```python
from build123d import *

# Parameters (mm, degrees)
EXTRUDE_1_DEPTH      = 5
EXTRUDE_1_DEPTH_BACK = 5
SKETCH_2_R           = 1.2
CUT_EXTRUDE_1_DEPTH  = 6
SKETCH_3_R           = 1.2
CUT_EXTRUDE_2_DEPTH  = 6
FILLET_1_R           = 1
FILLET_2_R           = 2
CUT_EXTRUDE1_DEPTH   = 2
CUT_EXTRUDE2_DEPTH   = 2


with BuildPart() as part:
    # Sketch 1 → Extrude 1 (new body, two sides)
    with BuildSketch(Plane(origin=(0, 0, 0), x_dir=(0, 0, -1), z_dir=(1, 0, 0))) as extrude_1_sk:
        Polygon((0, 44), (0, 0), (44, 0), (44, 5), (5, 5), (5, 44), align=None)
    extrude(amount=EXTRUDE_1_DEPTH)
    extrude(extrude_1_sk.sketch, amount=-EXTRUDE_1_DEPTH_BACK)

    # Sketch 2 → Cut-Extrude 1 (cut, through all)
    with BuildSketch(Plane(origin=(0, 5, 0), x_dir=(1, 0, 0), z_dir=(0, 1, 0))):
        with Locations((0, 39)):
            Circle(SKETCH_2_R)
        with Locations((0, 29)):
            Circle(SKETCH_2_R)
    extrude(amount=-CUT_EXTRUDE_1_DEPTH, mode=Mode.SUBTRACT)

    # Sketch 3 → Cut-Extrude 2 (cut, through all)
    with BuildSketch(Plane(origin=(0, 0, -5), x_dir=(-1, 0, 0), z_dir=(0, 0, -1))):
        with Locations((0, 39)):
            Circle(SKETCH_3_R)
        with Locations((0, 29)):
            Circle(SKETCH_3_R)
    extrude(amount=-CUT_EXTRUDE_2_DEPTH, mode=Mode.SUBTRACT)

    # Fillet 1
    fillet_1_edges = [part.edges().sort_by_distance(p)[0] for p in [
        (-5, 2.5, -44),
        (5, 44, -2.5),
        (5, 2.5, -44),
        (-5, 44, -2.5),
    ]]
    fillet(fillet_1_edges, radius=FILLET_1_R)

    # Fillet 2
    fillet_2_edges = [part.edges().sort_by_distance(p)[0] for p in [
        (0, 0, 0),
    ]]
    fillet(fillet_2_edges, radius=FILLET_2_R)

    # Sketch1 → Cut-Extrude1 (cut)
    with BuildSketch(Plane(origin=(0, 0, 0), x_dir=(-1, 0, 0), z_dir=(0, 0, -1))):
        Polygon((2, 27.845299462), (0, 26.690598923), (-2, 27.845299462), (-2, 30.154700538), (0, 31.309401077), (2, 30.154700538), align=None)
        Polygon((0, 41.309401077), (-2, 40.154700538), (-2, 37.845299462), (0, 36.690598923), (2, 37.845299462), (2, 40.154700538), align=None)
    extrude(amount=CUT_EXTRUDE1_DEPTH, mode=Mode.SUBTRACT)

    # Sketch2 → Cut-Extrude2 (cut)
    with BuildSketch(Plane(origin=(0, 0, 0), x_dir=(1, 0, 0), z_dir=(0, 1, 0))):
        Polygon((2.309401077, 29), (1.154700538, 31), (-1.154700538, 31), (-2.309401077, 29), (-1.154700538, 27), (1.154700538, 27), align=None)
        Polygon((1.154700538, 41), (2.309401077, 39), (1.154700538, 37), (-1.154700538, 37), (-2.309401077, 39), (-1.154700538, 41), align=None)
    extrude(amount=CUT_EXTRUDE2_DEPTH, mode=Mode.SUBTRACT)


solid = part.part
```
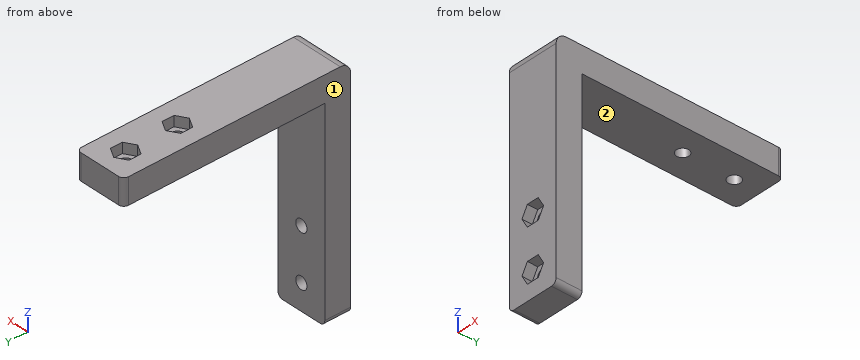
For this review, take the finished solid that the model builds, in its own axes (mm). Face numbers are marked on the shaded views. A direction names the side the tool comes from. Coordinates: 2 decimals unless noted, no trailing zeros. Write each loop counter-clockwise with the first axis right and the second up, starting at its lowest first coordinate (ties: lowest second). Pieces come first, ordered by that corner, then holes.
(1) Wall thickness on probe 1 along Y at (x, z) = (0, -2.7); probe 2 along Z at (x, y) = (0, 3.25); probe 3 along Y at (x, z) = (1.25, -40): over which ranges is each line inside the solid? List them lowest first.
(2) Tool access review of the marked faces 1 and 2: name each direction out of +Z, -Z, +X, -X, +Y, -Y from which nothing blocks a thin tool from reaching the whole face with its end or side.
(3) Add section A-A on y = 39. Give the boundary of the cut face in (x, z).
(4) For pin 1 Ø3 at (x, y) = (0, 29) entering from -Z; pin 2 Ø1.2 at (x, y) = (0, 29.5) entering from +Z; pin 3 Ø1.6 at (x, y) = (0, 0.5) entering from +Z; pin 4 Ø5 at (x, z) = (-1, -17.5) entering from +Y, all flat-tipped, find the tip position at first contact; note any pin that passes through.
(5) Add section B-B on y = 17.5. Give the boundary of the cut face in (x, z).
(6) Add section C-C on z = -16. Give the boundary of the cut face in (x, y).
Answer sheet:
1. probe 1: y = 0 to 27.8, 30.2 to 37.8, 40.2 to 44
1. probe 2: z = -44 to -40.2, -37.8 to -30.2, -27.8 to 0
1. probe 3: y = 2 to 5
2. face 1: +Z, -Z, -X, +Y, -Y
2. face 2: -Z, +X, -X, +Y
3. outline: (-5, -5) - (-1.2, -5) - (-1.2, -2) - (-2, -2) - (-2, 0) - (-5, 0) - close; (1.2, -5) - (5, -5) - (5, 0) - (2, 0) - (2, -2) - (1.2, -2) - close
4. pin 1: stops at z = -5
4. pin 2: passes through
4. pin 3: stops at z = -0.13
4. pin 4: stops at y = 5
5. outline: (-5, -5) - (5, -5) - (5, 0) - (-5, 0) - close
6. outline: (-5, 0) - (5, 0) - (5, 5) - (-5, 5) - close
